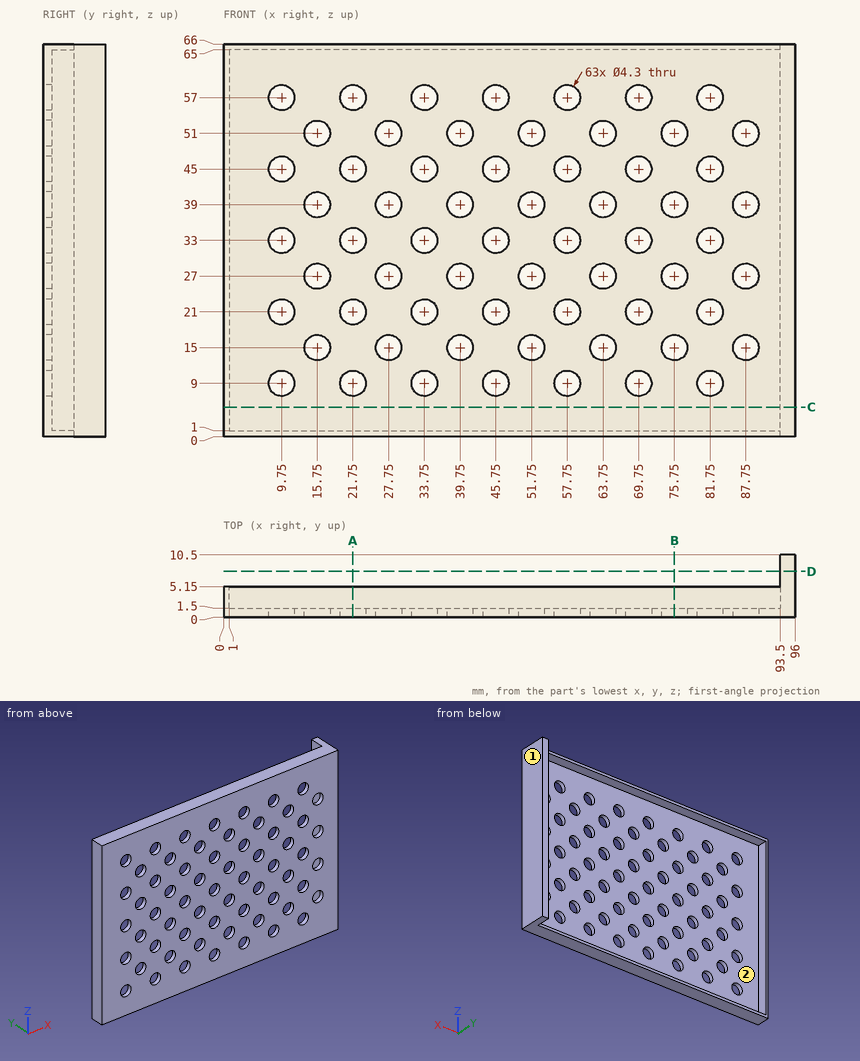
Geometry check sheet. Reference: drawing and pictorial views, mm from the part's lowest x, y, z. Coordinates: 2 decimals unless noted, no trailing zeros. Write each loop counter-clockwise with the first axis right and the second up, starting at its lowest first coordinate (ties: lowest second). Pieces come first, ordered by that corner, then holes.
Item 1: Scan lines: probe 1 along Z at (x, y) = (16, 0.5); probe 2 along Z at (x, y) = (9.75, 0.95); probe 3 along X at (y, z) = (4, 44). Record each from-to range of solid material in increasing order.
Numbers:
probe 1: z = 0 to 12.86, 17.14 to 24.86, 29.14 to 36.86, 41.14 to 48.86, 53.14 to 66
probe 2: z = 0 to 6.85, 11.15 to 18.85, 23.15 to 30.85, 35.15 to 42.85, 47.15 to 54.85, 59.15 to 66
probe 3: x = 0 to 1, 93.5 to 96
Item 2: Cross-section at B-B on x = 75.75. Record the boundary of the cut face in (y, z), then the cut area to 3 significant figures.
Numbers:
outline: (0, 0) - (5.15, 0) - (5.15, 1) - (1.5, 1) - (1.5, 12.85) - (0, 12.85) - close; (0, 17.15) - (1.5, 17.15) - (1.5, 24.85) - (0, 24.85) - close; (0, 29.15) - (1.5, 29.15) - (1.5, 36.85) - (0, 36.85) - close; (0, 41.15) - (1.5, 41.15) - (1.5, 48.85) - (0, 48.85) - close; (0, 53.15) - (1.5, 53.15) - (1.5, 65) - (5.15, 65) - (5.15, 66) - (0, 66) - close
area: 80.5 mm2
Item 3: Cross-section at C-C on z = 5. Record the boundary of the cut face in (x, y).
Numbers:
outline: (0, 0) - (96, 0) - (96, 10.5) - (93.5, 10.5) - (93.5, 1.5) - (1, 1.5) - (1, 5.15) - (0, 5.15) - close
Item 4: Cross-section at A-A on x = 21.75. Record the boundary of the cut face in (y, z), then the cut area to 4 significant figures.
Numbers:
outline: (0, 0) - (5.15, 0) - (5.15, 1) - (1.5, 1) - (1.5, 6.85) - (0, 6.85) - close; (0, 11.15) - (1.5, 11.15) - (1.5, 18.85) - (0, 18.85) - close; (0, 23.15) - (1.5, 23.15) - (1.5, 30.85) - (0, 30.85) - close; (0, 35.15) - (1.5, 35.15) - (1.5, 42.85) - (0, 42.85) - close; (0, 47.15) - (1.5, 47.15) - (1.5, 54.85) - (0, 54.85) - close; (0, 59.15) - (1.5, 59.15) - (1.5, 65) - (5.15, 65) - (5.15, 66) - (0, 66) - close
area: 74.05 mm2
Item 5: Depth check by flat-ended pin: pin 1 Ø3.5 at (x, z) = (21.75, 33) entering from -Y; pin 2 Ø3 at (y, z) = (7.5, 30.5) entering from -X; pin 3 Ø8 at (x, z) = (67, 23.5) entering from +Y. Enter the tip coordinate at first touch or a pass-through.
Numbers:
pin 1: passes through
pin 2: stops at x = 93.5
pin 3: stops at y = 1.5
Item 6: Cross-section at D-D on y = 7.75. Record the boundary of the cut face in (x, z), then the cut area to 3 significant figures.
Numbers:
outline: (93.5, 0) - (96, 0) - (96, 66) - (93.5, 66) - close
area: 165 mm2
Item 7: Mould release check, pull along Z, two halves, no side actions. Record for the marked faces 1 and 2: released by +Z, released by -Z, zero draft, split by the parting line, or undercut.
Numbers:
face 1: zero draft
face 2: undercut
